```python
from build123d import *

# Parameters (mm, degrees)
MODEL_R                 = 1.5
SALIENTE_EXTRUIR1_DEPTH = 3


with BuildPart() as part:
    # Model → Saliente-Extruir1 (new body)
    with BuildSketch(Plane.XY):
        with BuildLine():
            Line((174.227054575, 213.178720063), (174.227054575, 204.178720063))
            ThreePointArc((174.227054575, 204.178720063), (174.569596678, 202.456644617), (175.545074059, 200.996739548))
            Line((175.545074059, 200.996739548), (184.545074059, 191.996739548))
            ThreePointArc((184.545074059, 191.996739548), (187.727054575, 190.678720063), (190.90903509, 191.996739548))
            Line((190.90903509, 191.996739548), (199.90903509, 200.996739548))
            ThreePointArc((199.90903509, 200.996739548), (200.884512471, 202.456644617), (201.227054575, 204.178720063))
            Line((201.227054575, 204.178720063), (201.227054575, 235.678720063))
            Line((201.227054575, 235.678720063), (174.227054575, 235.678720063))
            Line((174.227054575, 235.678720063), (174.227054575, 213.178720063))
        make_face()
        with Locations((187.727054575, 204.178720063)):
            Circle(MODEL_R, mode=Mode.SUBTRACT)
        with Locations((178.727054575, 204.178720063)):
            Circle(MODEL_R, mode=Mode.SUBTRACT)
        with Locations((187.727054575, 213.178720063)):
            Circle(MODEL_R, mode=Mode.SUBTRACT)
        with Locations((178.727054575, 213.178720063)):
            Circle(MODEL_R, mode=Mode.SUBTRACT)
        with Locations((196.727054575, 213.178720063)):
            Circle(MODEL_R, mode=Mode.SUBTRACT)
        with Locations((187.727054575, 195.178720063)):
            Circle(MODEL_R, mode=Mode.SUBTRACT)
        with Locations((196.727054575, 204.178720063)):
            Circle(MODEL_R, mode=Mode.SUBTRACT)
        with Locations((187.727054575, 222.178720063)):
            Circle(MODEL_R, mode=Mode.SUBTRACT)
        with Locations((178.727054575, 222.178720063)):
            Circle(MODEL_R, mode=Mode.SUBTRACT)
        with Locations((196.727054575, 222.178720063)):
            Circle(MODEL_R, mode=Mode.SUBTRACT)
        with Locations((187.727054575, 231.178720063)):
            Circle(MODEL_R, mode=Mode.SUBTRACT)
        with Locations((178.727054575, 231.178720063)):
            Circle(MODEL_R, mode=Mode.SUBTRACT)
        with Locations((196.727054575, 231.178720063)):
            Circle(MODEL_R, mode=Mode.SUBTRACT)
    extrude(amount=SALIENTE_EXTRUIR1_DEPTH)


solid = part.part
```
Can you work these out from the model? Positions are in its coordinate system, mm. Give positions to 0.01 mm unless a question says otherwise; leave off trailing zeros. Loops run counter-clockwise (first coordinate to the right, second up) from the corner with the lowest first, then second, coordinate; pieces in that order, holes last. Notation, with made-up numbers: M 50,31 L 83,31 A22 ccw 83,45 Z; hole C 2.5,46.5 d7. An arc over 180 degrees is marked long. Use one line per item in the form item = value. Start each with the question number.
(1) I want a section at A-A, the plane x = 196.25. Write out the boundary of the cut face in (y, z).
(2) I'm going to push flat-ended pins straight in: P1, Ø2.5, axis at x = 178.73, y = 213.18, coming from the -Z side; P2, Ø1, axis at x = 196, z = 2.5, coming from the -Y side. Where does each tip first touch, or does it pass through?
(3) Please list where these lines run through material, in increasing order: line 1 (Y direction, x = 187.75, z = 2.85); line 2 (Y direction, x = 196, z = 1.5); line 3 (Y direction, x = 188.5, z = 1.2).
(4) Thinking about a two-plate mould opening in Y: for faces 1 (the cylindrical face through (187.68, 190.68, 1.48)), 2 (the cylindrical face through (188.533, 214.444, 1.479)), 3 (the cylindrical face through (197.533, 223.444, 1.479)), 4 (the flat face through (174.227, 220, 1)), which applies, released by +Y, released by -Y, zero draft, split by the parting line, or undercut?
(5) I want a section at C-C, the plane z = 1.65. State how many separate pieces and enclosed holes the cut face has, and give its area (3 significant figures).
(6) I want a section at B-B, the plane y = 221.5. Write out the boundary of the cut face in (x, z).
(7) I want a section at D-D, the plane x = 187.25. Write out the boundary of the cut face in (y, z), and give its area (3 significant figures).
Worked out:
q1.outline = M 197.34,0 L 202.76,0 L 202.76,3 L 197.34,3 Z; M 205.6,0 L 211.76,0 L 211.76,3 L 205.6,3 Z; M 214.6,0 L 220.76,0 L 220.76,3 L 214.6,3 Z; M 223.6,0 L 229.76,0 L 229.76,3 L 223.6,3 Z; M 232.6,0 L 235.68,0 L 235.68,3 L 232.6,3 Z
q2.P1 = through
q2.P2 = 196.59
q3.line_1 = 190.68 to 193.68, 196.68 to 202.68, 205.68 to 211.68, 214.68 to 220.68, 223.68 to 229.68, 232.68 to 235.68
q3.line_2 = 197.09 to 202.87, 205.49 to 211.87, 214.49 to 220.87, 223.49 to 229.87, 232.49 to 235.68
q3.line_3 = 190.75 to 193.89, 196.46 to 202.89, 205.46 to 211.89, 214.46 to 220.89, 223.46 to 229.89, 232.46 to 235.68
q4.face_1 = released by -Y
q4.face_2 = undercut
q4.face_3 = undercut
q4.face_4 = zero draft
q5.separate_pieces = 1
q5.enclosed_holes = 13
q5.area = 986 mm²
q6.outline = M 174.23,0 L 177.39,0 L 177.39,3 L 174.23,3 Z; M 180.06,0 L 186.39,0 L 186.39,3 L 180.06,3 Z; M 189.06,0 L 195.39,0 L 195.39,3 L 189.06,3 Z; M 198.06,0 L 201.23,0 L 201.23,3 L 198.06,3 Z
q7.outline = M 190.7,0 L 193.76,0 L 193.76,3 L 190.7,3 Z; M 196.6,0 L 202.76,0 L 202.76,3 L 196.6,3 Z; M 205.6,0 L 211.76,0 L 211.76,3 L 205.6,3 Z; M 214.6,0 L 220.76,0 L 220.76,3 L 214.6,3 Z; M 223.6,0 L 229.76,0 L 229.76,3 L 223.6,3 Z; M 232.6,0 L 235.68,0 L 235.68,3 L 232.6,3 Z
q7.area = 92.3 mm²
